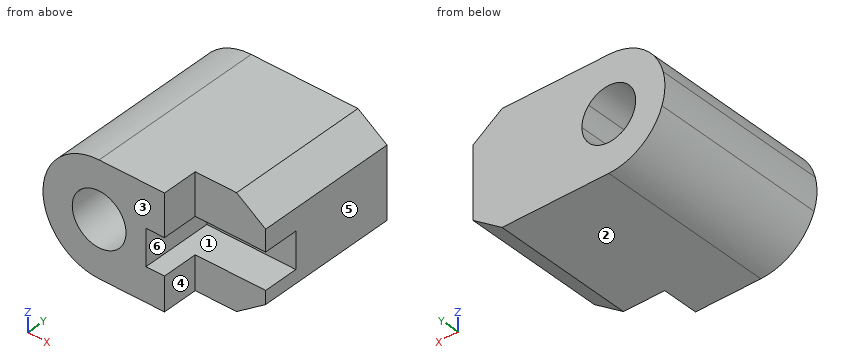
from build123d import *

# Parameters (mm, degrees)
F1_DEPTH = 25
F2_W     = 9.942237
F2_H     = 5.052494
F3_DEPTH = 15.773309
F4_W     = 10.188986
F4_H     = 5.094493
F5_DEPTH = 12.5


with BuildPart() as f1:
    # F0 (on Front) → F1 (new body)
    with BuildSketch(Plane.XZ):
        with BuildLine():
            Line((2.829923, 2.5), (7.479401, 2.5))
            ThreePointArc((7.479401, 2.5), (4.608473, 6.399485), (0, 7.886155))
            ThreePointArc((0, 7.886155), (-4.843936, 6.22316), (-7.64494, 1.935543))
            Line((-7.64494, 1.935543), (-3.242242, 1.935543))
            ThreePointArc((-3.242242, 1.935543), (-0.349506, 3.759828), (2.829923, 2.5))
        make_face()
        with BuildLine():
            Line((19.082905, 2.5), (7.479401, 2.5))
            Line((7.479401, 2.5), (2.829923, 2.5))
            ThreePointArc((2.829923, 2.5), (3.531597, 1.336519), (3.776038, 0))
            ThreePointArc((3.776038, 0), (3.531597, -1.336519), (2.829923, -2.5))
            Line((2.829923, -2.5), (7.479401, -2.5))
            Line((7.479401, -2.5), (19.082905, -2.5))
            Line((19.082905, -2.5), (19.082905, 2.5))
        make_face()
        with BuildLine():
            ThreePointArc((0, 7.886155), (4.608473, 6.399485), (7.479401, 2.5))
            Line((7.479401, 2.5), (19.082905, 2.5))
            Line((19.082905, 2.5), (19.082905, 5))
            Line((19.082905, 5), (15, 7.886155))
            Line((15, 7.886155), (0, 7.886155))
        make_face()
        with BuildLine():
            Line((-3.242242, 1.935543), (-7.64494, 1.935543))
            ThreePointArc((-7.64494, 1.935543), (-7.880668, -0.294115), (-7.479401, -2.5))
            ThreePointArc((-7.479401, -2.5), (-4.608473, -6.399485), (0, -7.886155))
            ThreePointArc((0, -7.886155), (4.608473, -6.399485), (7.479401, -2.5))
            Line((7.479401, -2.5), (2.829923, -2.5))
            ThreePointArc((2.829923, -2.5), (-2.227333, -3.049172), (-3.242242, 1.935543))
        make_face()
        with BuildLine():
            Line((19.082905, -5), (19.082905, -2.5))
            Line((19.082905, -2.5), (7.479401, -2.5))
            ThreePointArc((7.479401, -2.5), (4.608473, -6.399485), (0, -7.886155))
            Line((0, -7.886155), (15, -7.886155))
            Line((15, -7.886155), (19.082905, -5))
        make_face()
    extrude(amount=F1_DEPTH)

    # F2 (on face) → F3 (cut, through all)
    with BuildSketch(Plane.XY.offset(7.886155)):
        with Locations((14.159961, -22.473753)):
            Rectangle(F2_W, F2_H)
    extrude(amount=-F3_DEPTH, mode=Mode.SUBTRACT)

    # F4 (on face) → F5 (cut, symmetric)
    with BuildSketch(Plane.YZ.offset(19.082905)):
        with Locations((-20.086851, -0.580305)):
            Rectangle(F4_W, F4_H)
    extrude(amount=F5_DEPTH, both=True, mode=Mode.SUBTRACT)


solid = f1.part
Read the model definition and answer for the solid it produces. Units are mm, in the model's axes. Face numbers are marked on the shaded views. A direction names the side the tool comes from. Give positions to 0.01 mm unless a question says otherwise; leave off trailing zeros. Write each loop counter-clockwise with the first axis right and the second up, starting at its lowest first coordinate (ties: lowest second). Pieces come first, ordered by that corner, then holes. Notation, with made-up numbers: (-38.75, -5.75) -> (16.25, -5.75) arc R28 ccw to (16.25, 24.25) -> close; hole circle Ø5 at (50, 43.25). An arc over 180 degrees is marked (long way). Answer as a JSON object with one key per item and string values. Group by question number.
1) Find section B-B (x = 1.75). Write down the section's boundary in (y, z), and give its area (3 significant figures).
2) A tool of negligible diameter and unlimited length cuts with its end or side. For the marked faces 4, 5 and 6, from which of +Z, -Z, +X, -X, +Y, -Y can it reach the whole face along a straight path? Write none if from no direction.
3) Consider L1, parallel to Z at x = -0.25, y = -3; L2, parallel to Y at x = 16.25, z = -6; L3, parallel to X at y = -17.25, z = -0.25. Determine where each line is inside the solid, lowest interval first. Write a range as from..to.
4) Each of these flat-tipped pins is pushed along its axis until it touches: P1, Ø4.5, axis at x = 12.5, z = 4, coming from the -Y side; P2, Ø3, axis at x = 15, y = -21.5, coming from the +Z side; P3, Ø1.5, axis at x = 8.5, z = -1.5, coming from the -Y side; P4, Ø1.5, axis at y = -21.5, z = 5.5, coming from the +X side. Where does it stop, or does it pass through?
5) The mould has two halves that part along Z. Classify the marked faces 1, 2 and 3: +Z half, -Z half, draft (parallel to the pull), parting line (faces both ways), or undercut.
6) Find section C-C (x = 12.5). Write down the section's boundary in (y, z).
7) Find section A-A (y = -7). Write down the section's boundary in (x, z), and give its area (3 significant figures).
8) Find section D-D (y = -17.25). Write down the section's boundary in (x, z), and give its area (3 significant figures).
Values follow:
{
 "1": {"outline": "(-25, -7.89) -> (0, -7.89) -> (0, -3.35) -> (-25, -3.35) -> close; (-25, 3.35) -> (0, 3.35) -> (0, 7.89) -> (-25, 7.89) -> close", "area": "227 mm2"},
 "2": {"face 4": "+Z, -Z, +X, -Y", "face 5": "+Z, -Z, +X, +Y, -Y", "face 6": "+X, -Y"},
 "3": {"L1": "z = -7.88..-3.77, 3.77..7.88", "L2": "y = -19.95..0", "L3": "x = -7.88..-3.77, 3.77..6.58"},
 "4": {"P1": "stops at y = -19.95", "P2": "passes through", "P3": "stops at y = -14.99", "P4": "stops at x = 9.19"},
 "5": {"face 1": "undercut", "face 2": "-Z half", "face 3": "draft"},
 "6": {"outline": "(-19.95, -7.89) -> (0, -7.89) -> (0, 7.89) -> (-19.95, 7.89) -> (-19.95, 1.97) -> (-14.99, 1.97) -> (-14.99, -3.13) -> (-19.95, -3.13) -> close"},
 "7": {"outline": "(-7.64, 1.94) arc R7.89 ccw to (-7.48, -2.5) arc R7.89 ccw to (0, -7.89) -> (15, -7.89) -> (19.08, -5) -> (19.08, 5) -> (15, 7.89) -> (0, 7.89) arc R7.89 ccw to start; hole (2.83, -2.5) arc R3.78 ccw to (3.78, 0) arc R3.78 ccw to (2.83, 2.5) arc R3.78 ccw (long way) to start", "area": "342 mm2"},
 "8": {"outline": "(-7.64, 1.94) arc R7.89 ccw to (-7.48, -2.5) arc R7.89 ccw to (0, -7.89) -> (15, -7.89) -> (19.08, -5) -> (19.08, -3.13) -> (6.58, -3.13) -> (6.58, 1.97) -> (19.08, 1.97) -> (19.08, 5) -> (15, 7.89) -> (0, 7.89) arc R7.89 ccw to start; hole (2.83, -2.5) arc R3.78 ccw to (3.78, 0) arc R3.78 ccw to (2.83, 2.5) arc R3.78 ccw (long way) to start", "area": "278 mm2"}
}
